```python
from build123d import *

# Parameters (mm, degrees)
SKETCH1_R                 = 19
SKETCH1_R_2               = 14
BOSS_EXTRUDE1_DEPTH       = 125
BOSS_EXTRUDE2_START       = 7.5
SKETCH2_R                 = 14
BOSS_EXTRUDE2_DEPTH       = 7.5
CUT_EXTRUDE1_DEPTH        = 121.53319045
CUT_EXTRUDE1_DEPTH_BACK   = 121.53319045
SKETCH4_R                 = 6.025
SKETCH5_R                 = 14
BOSS_EXTRUDE3_DEPTH       = 7.5
BOSS_EXTRUDE4_DEPTH       = 15
BOSS_EXTRUDE4_DEPTH_BACK  = 140
SKETCH7_R                 = 6.025
SKETCH8_R                 = 15
BOSS_EXTRUDE5_DEPTH       = 5
LPATTERN2_COUNT           = 2
LPATTERN2_PITCH           = 30
LPATTERN3_COPY_1_SKETCH_R = 15
LPATTERN3_COPY_1_DEPTH    = 5
LPATTERN3_COPY_2_SKETCH_R = 15
LPATTERN3_COPY_2_DEPTH    = 5


with BuildPart() as part:
    # Sketch1 → Boss-Extrude1 (new body)
    with BuildSketch(Plane.XY):
        Circle(SKETCH1_R)
        Circle(SKETCH1_R_2, mode=Mode.SUBTRACT)
    extrude(amount=-BOSS_EXTRUDE1_DEPTH)

    # Sketch2 → Boss-Extrude2 (add)
    with BuildSketch(Plane.XY.offset(-7.5).offset(BOSS_EXTRUDE2_START)):
        Circle(SKETCH2_R)
    extrude(amount=-BOSS_EXTRUDE2_DEPTH)

    # Sketch4 → Cut-Extrude1 (cut, two sides: drawn at the far end of the back side and taken through both)
    with BuildSketch(Plane.XY.offset(-7.5).offset(-CUT_EXTRUDE1_DEPTH_BACK)):
        Circle(SKETCH4_R)
    extrude(amount=CUT_EXTRUDE1_DEPTH + CUT_EXTRUDE1_DEPTH_BACK, mode=Mode.SUBTRACT)

    # Sketch5 → Boss-Extrude3 (add)
    with BuildSketch(Plane(origin=(0, 0, -117.5), x_dir=(-1, 0, 0), z_dir=(0, 0, -1))):
        with Locations(Location((0, 0, 0), (0, 0, 180))):
            Circle(SKETCH5_R)
    extrude(amount=BOSS_EXTRUDE3_DEPTH)

    # Sketch7 → Boss-Extrude4 (add, two sides: drawn at the far end of the back side and taken through both)
    with BuildSketch(Plane.XY.offset(-BOSS_EXTRUDE4_DEPTH_BACK)):
        Circle(SKETCH7_R)
    extrude(amount=BOSS_EXTRUDE4_DEPTH + BOSS_EXTRUDE4_DEPTH_BACK)

    # Sketch8 → Boss-Extrude5 (add, symmetric)
    with BuildSketch(Plane.XY.offset(-62.5)):
        Circle(SKETCH8_R)
    boss_extrude5 = extrude(amount=BOSS_EXTRUDE5_DEPTH, both=True)

    # LPattern2: Boss-Extrude5 ×2
    with Locations(*[(0, 0, -i * LPATTERN2_PITCH) for i in range(1, LPATTERN2_COUNT)]):
        add(boss_extrude5)

    # LPattern3 copy 1 sketch → LPattern3 copy 1 (add, symmetric)
    with BuildSketch(Plane.XY.offset(-62.5)):
        Circle(LPATTERN3_COPY_1_SKETCH_R)
    extrude(amount=LPATTERN3_COPY_1_DEPTH, both=True)

    # LPattern3 copy 2 sketch → LPattern3 copy 2 (add, symmetric)
    with BuildSketch(Plane.XY.offset(-32.5)):
        Circle(LPATTERN3_COPY_2_SKETCH_R)
    extrude(amount=LPATTERN3_COPY_2_DEPTH, both=True)


solid = part.part
```
Work out the finished part from the listing and answer in its coordinate system (mm). A direction names the side the tool comes from. Coordinates: 2 decimals unless noted, no trailing zeros. Order: outer loops, then holes, each group sorted by start corner. A loop starts at its lowest first (then second) coordinate and runs counter-clockwise, first axis right, second up. Notation, with made-up numbers: (55, -26.5) - (110, -26.5) arc R6 cw to (110, -22.5) - close; hole circle Ø5 at (70.5, 23). An arc over 180 degrees is marked (long way). Answer as a JSON object with one key per item and string values.
1. Find section D-D on y = 0. Count the separate pieces of the cut face and the enclosed holes in it, plus the area to 3 significant figures.
Output values:
{"separate pieces": "1", "enclosed holes": "8", "area": "3,840 mm²"}
2. Find section B-B on x = 10.5. Determine the outline of the cut face in (y, z).
Output values:
{"outline": "(-15.84, -125) - (15.84, -125) - (15.84, 0) - (-15.84, 0) - close; hole (-9.26, -117.5) - (9.26, -117.5) - (9.26, -97.5) - (-9.26, -97.5) - close; hole (-9.26, -87.5) - (9.26, -87.5) - (9.26, -67.5) - (-9.26, -67.5) - close; hole (-9.26, -57.5) - (9.26, -57.5) - (9.26, -37.5) - (-9.26, -37.5) - close; hole (-9.26, -27.5) - (9.26, -27.5) - (9.26, -7.5) - (-9.26, -7.5) - close"}
3. Find section A-A on y = 11. Determine the outline of the cut face in (x, z), plus the area to 3 significant figures.
Output values:
{"outline": "(-15.49, -125) - (15.49, -125) - (15.49, 0) - (-15.49, 0) - close; hole (-8.66, -117.5) - (8.66, -117.5) - (8.66, -97.5) - (-8.66, -97.5) - close; hole (-8.66, -87.5) - (8.66, -87.5) - (8.66, -67.5) - (-8.66, -67.5) - close; hole (-8.66, -57.5) - (8.66, -57.5) - (8.66, -37.5) - (-8.66, -37.5) - close; hole (-8.66, -27.5) - (8.66, -27.5) - (8.66, -7.5) - (-8.66, -7.5) - close", "area": "2,490 mm²"}
4. Find section C-C on z = -26. Determine the outline of the cut face in (x, y) (3 decimals), plus the area to 3 significant figures.
Output values:
{"outline": "circle Ø38 at (0, 0); circle Ø12.05 at (0, 0); hole circle Ø28 at (0, 0)", "area": "632 mm²"}
5. Consider line 1 (Y direction, x = 0, z = -103) (3 decimals); line 2 (Z direction, x = -11.5, y = 7); line 3 (X direction, y = 4, z = -101.5). Determine where each line is inside the solid, lowest interval first.
Output values:
{"line 1": "y = -19 to -14, -6.025 to 6.025, 14 to 19", "line 2": "z = -125 to -117.5, -97.5 to -87.5, -67.5 to -57.5, -37.5 to -27.5, -7.5 to 0", "line 3": "x = -18.57 to -13.42, -4.51 to 4.51, 13.42 to 18.57"}
6. The mould has two halves that part along Z. Classify faces 5 (the face through (-4.44, 4.07, 7.4)), 6 (the face through (-4.44, 4.07, -107.64)), 7 (the face through (0, 0, 15)): +Z half, -Z half, draft (parallel to the pull), parting line (faces both ways), or undercut.
Output values:
{"face 5": "draft", "face 6": "undercut", "face 7": "+Z half"}
7. Each of these flat-tipped pins is pushed along its axis until it touches: P1, Ø2, axis at x = 1.5, z = -37, coming from the -Y side; P2, Ø10, axis at y = 14.5, z = -29.5, coming from the +X side; P3, Ø2, axis at x = -12, y = -1.5, coming from the -Z side. Where does it stop, or does it pass through?
Output values:
{"P1": "stops at y = -18.99", "P2": "stops at x = 16.45", "P3": "stops at z = -125"}
8. A tool of negligible diameter and unlimited length cuts with its end or side. For faces 1 (the face through (-4.44, 4.07, -132.6)), 2 (the face through (8.767, -16.856, -61.625)), 3 (the face through (-4.5, 4.5, 0)), 4 (the face through (-4.44, 4.07, -47.64)), from which of +Z, -Z, +X, -X, +Y, -Y can it reach the whole face along a straight path? Write none if from no direction.
Output values:
{"face 1": "-Z", "face 2": "+Z, -Z", "face 3": "+Z", "face 4": "none"}
